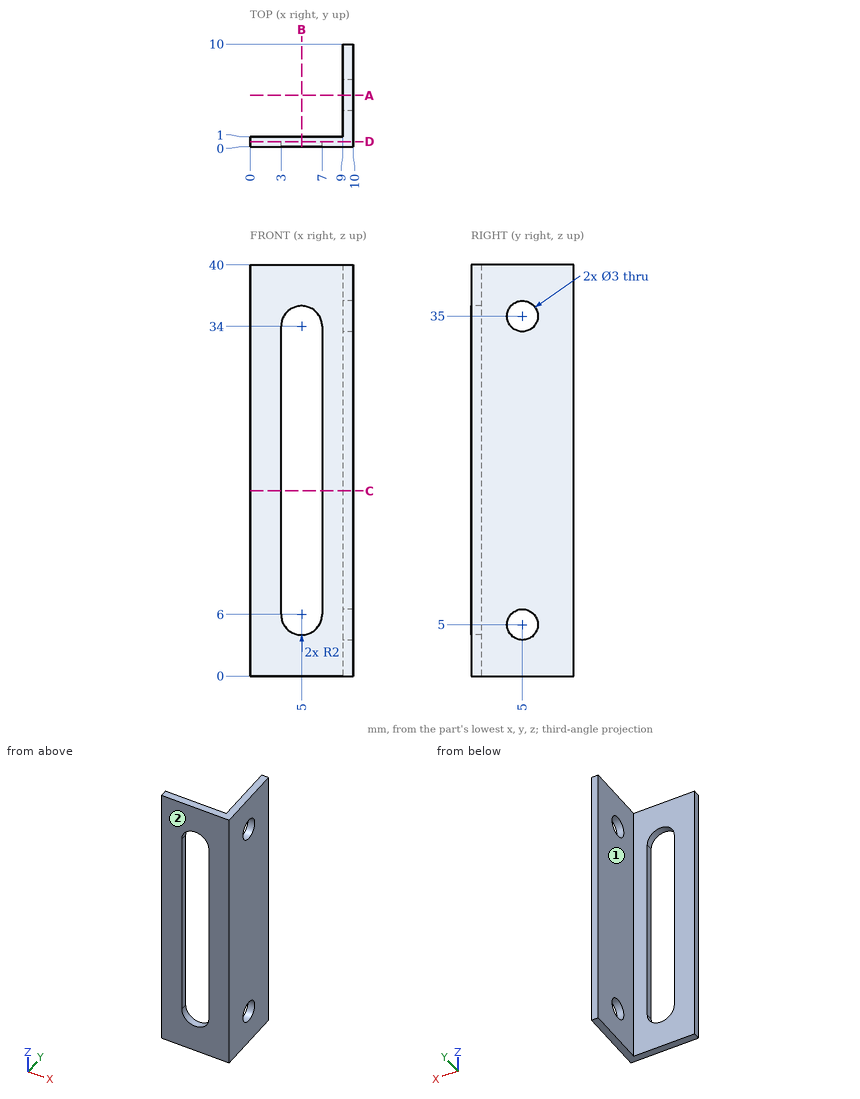
Drawing for the job (mm, zero at the part's lowest x, y, z). A direction names the side the tool comes from. Round coordinates to 2 decimals unless told otherwise and drop trailing zeros. Loops run counter-clockwise (first coordinate to the right, second up) from the corner with the lowest first, then second, coordinate; pieces in that order, holes last.
1. Band-saw the part on A-A, the plane y = 5. List the corners of the cut face in (x, z), and give its area (3 significant figures).
Check values:
outline: (9, 0) - (10, 0) - (10, 3.5) - (9, 3.5) - close; (9, 6.5) - (10, 6.5) - (10, 33.5) - (9, 33.5) - close; (9, 36.5) - (10, 36.5) - (10, 40) - (9, 40) - close
area: 34.0 mm2
2. Drop flat-ended pins along their axis: P1, Ø3, axis at x = 5, z = 29.5, coming from the +Y side; P2, Ø1, axis at y = 7, z = 13.5, coming from the -X side. Give the stop position or say it passes through.
Check values:
P1: passes through
P2: stops at x = 9
3. Band-saw the part on B-B, the plane x = 5. List the corners of the cut face in (y, z), and give its area (3 significant figures).
Check values:
outline: (0, 0) - (1, 0) - (1, 4) - (0, 4) - close; (0, 36) - (1, 36) - (1, 40) - (0, 40) - close
area: 8.00 mm2
4. Tool access for the marked faces 1 and 2: list every direction of +Z, -Z, +X, -X, +Y, -Y with a clear straight run to the whole face (end or side of a thin tool).
Check values:
face 1: +Z, -Z, -X, +Y
face 2: +Z, -Z, +X, -X, -Y
5. Wall check: probe 1 along Z at (x, y) = (9.55, 5); probe 2 along Y at (x, z) = (9.3, 35); probe 3 along X at (y, z) = (6, 30.5). Give the ranges that are in metal, low to high.
Check values:
probe 1: z = 0 to 3.5, 6.5 to 33.5, 36.5 to 40
probe 2: y = 0 to 3.5, 6.5 to 10
probe 3: x = 9 to 10
6. Band-saw the part on C-C, the plane z = 18. List the corners of the cut face in (x, y), and give its area (3 significant figures).
Check values:
outline: (0, 0) - (3, 0) - (3, 1) - (0, 1) - close; (7, 0) - (10, 0) - (10, 10) - (9, 10) - (9, 1) - (7, 1) - close
area: 15.0 mm2
7. Band-saw the part on D-D, the plane y = 0.5. List the corners of the cut face in (x, z), and give its area (3 significant figures).
Check values:
outline: (0, 0) - (10, 0) - (10, 40) - (0, 40) - close; hole (3, 6) arc R2 ccw to (7, 6) - (7, 34) arc R2 ccw to (3, 34) - close
area: 275 mm2
